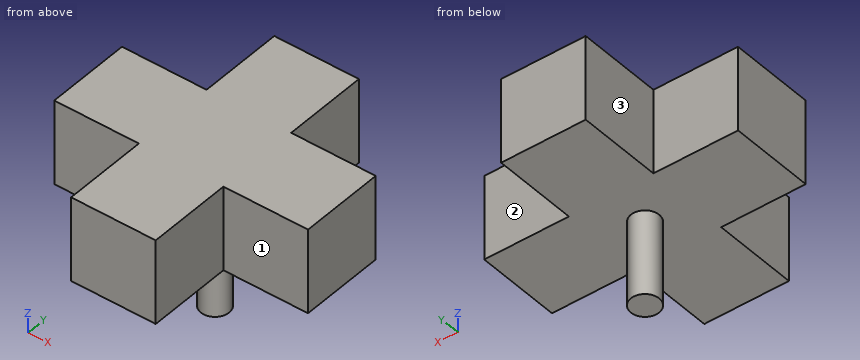
```python
from build123d import *

# Parameters (mm, degrees)
F1_DEPTH = 30
F2_R     = 5
F3_DEPTH = 30


with BuildPart() as f1:
    # F0 (on Top) → F1 (new body)
    with BuildSketch(Plane.XY):
        Polygon((45, -15), (45, 0), (45, 15), (15, 15), (15, 45), (0, 45), (-15, 45), (-15, 15), (-45, 15), (-45, 0), (-45, -15), (-15, -15), (-15, -45), (0, -45), (15, -45), (15, -15), align=None)
    extrude(amount=F1_DEPTH)

    # F2 (on face) → F3 (join)
    with BuildSketch(Plane(origin=(0, 0, 0), x_dir=(1, 0, 0), z_dir=(0, 0, -1))):
        Circle(F2_R)
    extrude(amount=F3_DEPTH)


solid = f1.part
```
For this review, take the finished solid that the model builds, in its own axes (mm). Face numbers are marked on the shaded views. A direction names the side the tool comes from. Give positions to 0.01 mm unless a question says otherwise; leave off trailing zeros. Loops run counter-clockwise (first coordinate to the right, second up) from the corner with the lowest first, then second, coordinate; pieces in that order, holes last. Notation, with made-up numbers: M -20.75,-4.5 L 18.25,-4.5 A24 ccw 18.25,16.5 Z; hole C 51.25,12 d5. An arc over 180 degrees is marked long. One line per item, written item: value. Start each with the question number.
Q1. For L1, parallel to X at y = -38.5, z = 25; L2, parallel to Z at x = 5.5, y = 31, list the stretches that pass through material, from the lowest coordinate up.
Q2. Clearance check with flat-ended pins moving along their axes: pin 1 Ø4 at (x, y) = (-15.5, -31.5) entering from -Z; pin 2 Ø24 at (x, z) = (-36.5, 10) entering from -Y; pin 3 Ø4 at (x, z) = (27.5, 3.5) entering from +Y. State where each tip first meets the part, or that it passes through.
Q3. Add section A-A (y = 0). Give the boundary of the cut face in (x, z), and give its area (3 significant figures).
Q4. Add section D-D (y = -31). Give the boundary of the cut face in (x, z), and give its area (3 significant figures).
Q5. Machinability: for the marked faces 1, 2 and 3, which of the approach directions +Z, -Z, +X, -X, +Y, -Y give a long, thin tool a straight path to every point of the face, cutting with its end or side? Answer none if there is none.
Q6. Add section B-B (z = 19.5). Give the boundary of the cut face in (x, y).
Reply:
1. L1: -15 to 15
1. L2: 0 to 30
2. pin 1: z = 0
2. pin 2: y = -15
2. pin 3: y = 15
3. outline: M -45,0 L -5,0 L -5,-30 L 5,-30 L 5,0 L 45,0 L 45,30 L -45,30 Z
3. area: 3,000 mm²
4. outline: M -15,0 L 15,0 L 15,30 L -15,30 Z
4. area: 900 mm²
5. face 1: +Z, -Z, +X, -Y
5. face 2: +Z, -Z, +X, +Y
5. face 3: +Z, -Z, -X, +Y
6. outline: M -45,-15 L -15,-15 L -15,-45 L 15,-45 L 15,-15 L 45,-15 L 45,15 L 15,15 L 15,45 L -15,45 L -15,15 L -45,15 Z
